Build history of the part. All positions in model axes, mm. A direction names the side the tool comes from. Round coordinates to 2 decimals unless told otherwise and drop trailing zeros. Loops run counter-clockwise (first coordinate to the right, second up) from the corner with the lowest first, then second, coordinate; pieces in that order, holes last. Notation, with made-up numbers: (32.5, -14.5) - (77.5, -14.5) arc R34 ccw to (77.5, 19.5) - close; hole circle Ø6 at (79.5, 21.25). An arc over 180 degrees is marked (long way). Put each result on its own line as item: value. Start each with the question number.
Autodesk Inventor part; units mm, degrees
ref_plane "YZ Plane" through (0, 0, 0) normal (1, 0, 0) x (0, 1, 0)
ref_plane "XZ Plane" through (0, 0, 0) normal (0, 1, 0) x (-1, 0, 0)
ref_plane "XY Plane" through (0, 0, 0) normal (0, 0, 1) x (1, 0, 0)
sketch "Эскиз1" plane through (0, 0, 0) normal (0, 1, 0) x (-1, 0, 0)
  circle A0 centre (0, 0) radius 9.5
  dimension "d0" = 19
extrude "Выдавливание1" add sketch "Эскиз1" along normal blind 25
sketch "Эскиз2" plane through (0, 25, 0) normal (0, 1, 0) x (1, 0, 0)
  circle A0 centre (0, 0) radius 4
  dimension "d3" = 8
extrude "Выдавливание2" cut sketch "Эскиз2" against normal blind 12.5
sketch "Эскиз3" plane through (0, 0, 0) normal (0, -1, 0) x (1, 0, 0)
  circle A0 centre (0, 0) radius 2.5
  dimension "d6" = 5
extrude "Выдавливание3" cut sketch "Эскиз3" against normal through all
thread "Резьба1"
chamfer "Фаска1" distance 0.5 angle 45 4 edges at (-4, 25, 0) (9.5, 25, 0) (9.5, 0, 0) (-2.5, 0, 0)
properties part number "mufta_5x8"
1) Slice it at D-D, the plane y = 11.25. Write the cut outline in (x, z).
2) Drop flat-ended pins along their axis: pin 1 Ø3 at (y, z) = (17, 7) entering from +X; pin 2 Ø1.5 at (x, z) = (4.5, -2.5) entering from -Y; pin 3 Ø1 at (y, z) = (3, 6.5) entering from +X; pin 4 Ø6 at (x, z) = (0, 0) entering from +Y. Give the stop position or say it passes through.
3) Pull direction X, two halves, no side cores. Call faces 1 (the face through (-4.38, 12.33, 8.43)), 2 (the face through (2, 12.5, -2)), 3 (the face through (-0.54, 6.42, -2.44)), 4 (the face through (-4, 25, -4)): pulls with the +X half, pulls with the -X half, needs draft (parallel to the pull), parting line crosses it, or undercut.
4) Slice it at B-B, the plane x = 0. Write the cut outline in (y, z).
5) Slice it at C-C, the plane y = 18. Write the cut outline in (x, z), and give its area (3 significant figures).
6) Slice it at A-A, the plane z = 0. Write the cut outline in (x, y).
7) Drill centre lines: line 1 (Z direction, x = 0, y = 4); line 2 (Z direction, x = -0.25, y = 23.25); line 3 (X direction, y = 13.5, z = -2.5). Where is each one in solid material? Low to high. Write a range as [from, to].
8) Which spindle directions (+Z, -Z, +X, -X, +Y, -Y) get a long thin tool onto all of the face, cutting with end or side? Do faces 5 (the face through (-0.867, 18.584, 3.905)), 6 (the face through (0, 0, -4)). Say none if no direction does.
Taken from the geometry:
1. outline: circle Ø19 at (0, 0); hole circle Ø5 at (0, 0)
2. pin 1: stops at x = 7.75
2. pin 2: stops at y = 0
2. pin 3: stops at x = 7.37
2. pin 4: stops at y = 12.5
3. face 1: parting line crosses it
3. face 2: undercut
3. face 3: undercut
3. face 4: needs draft
4. outline: (0, -9) - (0.5, -9.5) - (24.5, -9.5) - (25, -9) - (25, -4.5) - (24.5, -4) - (12.5, -4) - (12.5, -2.5) - (0.5, -2.5) - (0, -3) - close; (0, 3) - (0.5, 2.5) - (12.5, 2.5) - (12.5, 4) - (24.5, 4) - (25, 4.5) - (25, 9) - (24.5, 9.5) - (0.5, 9.5) - (0, 9) - close
5. outline: circle Ø19 at (0, 0); hole circle Ø8 at (0, 0)
5. area: 233 mm2
6. outline: (-9.5, 0.5) - (-9, 0) - (-3, 0) - (-2.5, 0.5) - (-2.5, 12.5) - (-4, 12.5) - (-4, 24.5) - (-4.5, 25) - (-9, 25) - (-9.5, 24.5) - close; (2.5, 0.5) - (3, 0) - (9, 0) - (9.5, 0.5) - (9.5, 24.5) - (9, 25) - (4.5, 25) - (4, 24.5) - (4, 12.5) - (2.5, 12.5) - close
7. line 1: z = [-9.5, -2.5], [2.5, 9.5]
7. line 2: z = [-9.5, -3.99], [3.99, 9.5]
7. line 3: x = [-9.17, -3.12], [3.12, 9.17]
8. face 5: +Y
8. face 6: +Z, -Z, +X, -X, -Y
